The drawing under review shows one solid part. Ordinate dimensions are in mm from its lowest x, y, z. Coordinates: 2 decimals unless noted, no trailing zeros. Order: outer loops, then holes, each group sorted by start corner. A loop starts at its lowest first (then second) coordinate and runs counter-clockwise, first axis right, second up. Notation, with made-up numbers: (-15, -34.5) -> (10, -34.5) arc R18 cw to (10, -21.5) -> close; hole circle Ø11 at (1.25, 49.5). An arc over 180 degrees is marked (long way). Use a Markdown table: item, result. Add a question column.
Q1. Wall thickness on probe 1 along Z at (x, y) = (13.5, 36.5); probe 2 along X at (y, z) = (30, 50); probe 3 along Z at (x, y) = (96, 31): over which ranges is each line inside the solid? List them lowest first.
Q2. Add section C-C (z = 50). State the section outline as (x, y) points.
Q3. Add section B-B (y = 44.5). State the section outline as (x, z) points.
Q4. The part is to be moulded in two halves that separate along X. For the marked faces 1, 2 and 3, say which applies: pulls with the +X half, pulls with the -X half, needs draft (parallel to the pull), parting line crosses it, or undercut.
Q5. Add section A-A (x = 13.5). State the section outline as (y, z) points.
Q6. Insertion check: pin 1 (3 mm diameter, centred on x = 13.5, z = 30.5, fed in from -Y). The pin has a flat end and moves straight along its axis. Give the tip position at first contact, or say it passes through.
Q7. Add section D-D (x = 55). State the section outline as (y, z) points, then the cut area to 3 significant figures.
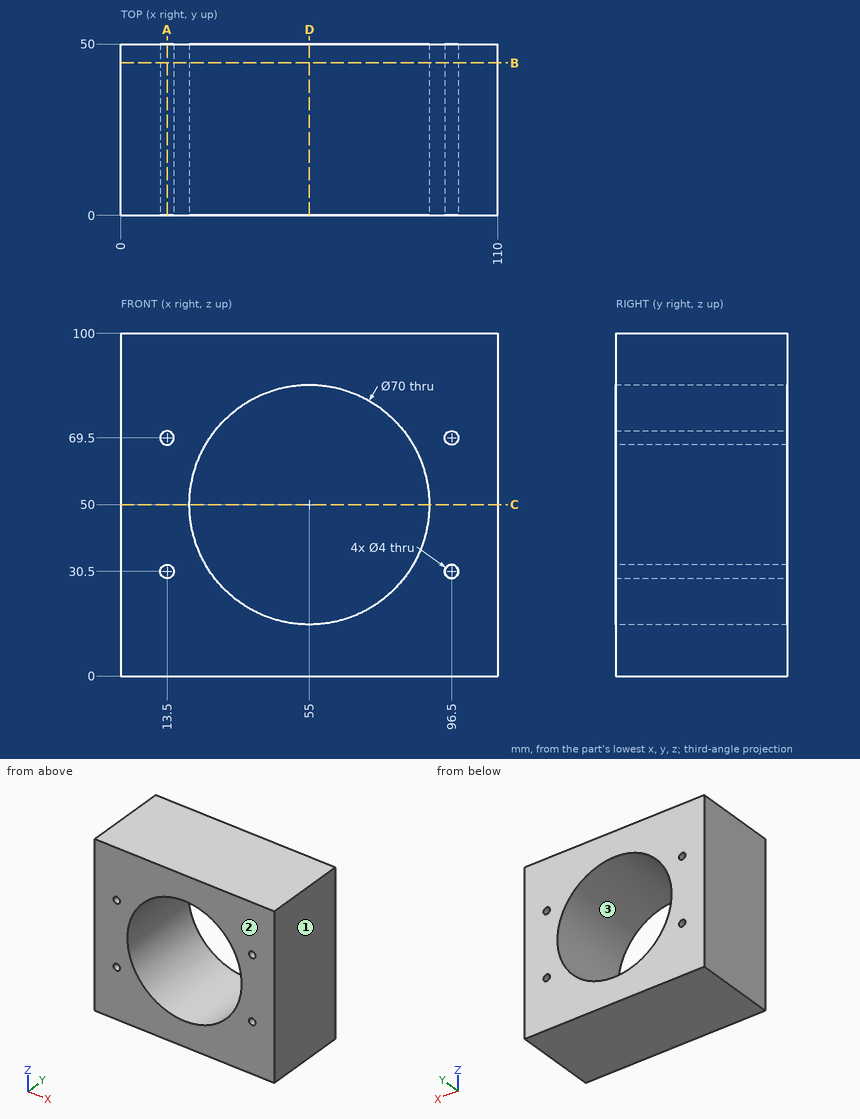
Established:
| question | item | result |
|---|---|---|
| 1 | probe 1 | 0 to 28.5, 32.5 to 67.5, 71.5 to 100 |
| 1 | probe 2 | 0 to 20, 90 to 110 |
| 1 | probe 3 | 0 to 28.56, 32.44 to 67.56, 71.44 to 100 |
| 2 | outline | (0, 0) -> (20, 0) -> (20, 50) -> (0, 50) -> close; (90, 0) -> (110, 0) -> (110, 50) -> (90, 50) -> close |
| 3 | outline | (0, 0) -> (110, 0) -> (110, 100) -> (0, 100) -> close; hole circle Ø4 at (13.5, 30.5); hole circle Ø4 at (13.5, 69.5); hole circle Ø70 at (55, 50); hole circle Ø4 at (96.5, 30.5); hole circle Ø4 at (96.5, 69.5) |
| 4 | face 1 | pulls with the +X half |
| 4 | face 2 | needs draft |
| 4 | face 3 | undercut |
| 5 | outline | (0, 0) -> (50, 0) -> (50, 28.5) -> (0, 28.5) -> close; (0, 32.5) -> (50, 32.5) -> (50, 67.5) -> (0, 67.5) -> close; (0, 71.5) -> (50, 71.5) -> (50, 100) -> (0, 100) -> close |
| 6 | pin 1 | through |
| 7 | outline | (0, 0) -> (50, 0) -> (50, 15) -> (0, 15) -> close; (0, 85) -> (50, 85) -> (50, 100) -> (0, 100) -> close |
| 7 | area | 1,500 mm^2 |
